Work out the finished part from the listing and answer in its coordinate system (mm). Face numbers are marked on the shaded views. A direction names the side the tool comes from. Coordinates: 2 decimals unless noted, no trailing zeros. Order: outer loops, then holes, each group sorted by start corner. A loop starts at its lowest first (then second) coordinate and runs counter-clockwise, first axis right, second up. Notation, with made-up numbers: (1.5, 54.5) - (20.5, 54.5) arc R13 cw to (20.5, 64.5) - close; hole circle Ø10 at (-20, 62.25). An arc over 180 degrees is marked (long way). Answer as a JSON object with one key per item and string values. Group by question number.
1) Section B-B (x = 2) is taken. Give the vertices of the cut face in (y, z).
2) Each of these flat-tipped pins is pushed along its axis until it touches: P1, Ø0.9, axis at x = -8.5, y = 1, coming from the -Z side; P2, Ø1, axis at x = 4, z = 2, coming from the -Y side; P3, Ø0.9, axis at x = -8.5, y = 0.5, coming from the +Z side. Where does it stop, or does it pass through?
3) Section C-C (y = 1) is taken. Give the vertices of the cut face in (x, z), plus the area to 3 significant figures.
4) A tool of negligible diameter and unlimited length cuts with its end or side. For the marked faces 1 and 2, from which of +Z, -Z, +X, -X, +Y, -Y can it reach the whole face along a straight path? Write none if from no direction.
5) Section A-A (y = 4.25) is taken. Give the vertices of the cut face in (x, z), plus the area to 3 significant figures.
6) Find the intervals of material crossed by line 1 along Z through (x, y) = (1.25, 1.25); line 2 along Z through (x, y) = (6.75, 2); line 3 along Y through (x, z) = (-5.25, 6.25), in increasing order.
7) Section D-D (z = 0.5) is taken. Give the vertices of the cut face in (x, y), plus the area to 3 significant figures.
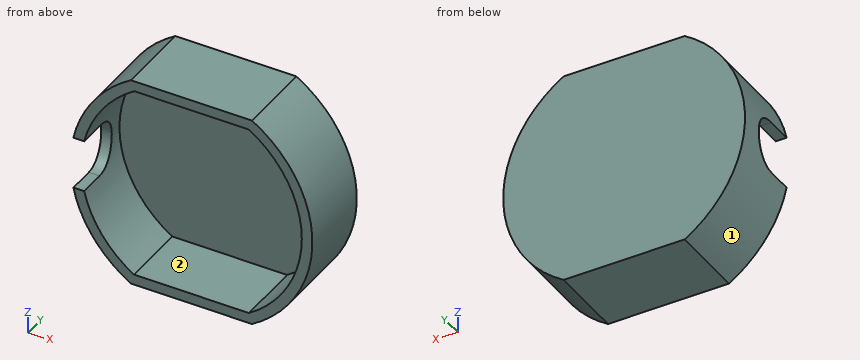
from build123d import *

# Parameters (mm, degrees)
BOSS_EXTRUDE1_DEPTH = 5
BOSS_EXTRUDE2_DEPTH = 0.8
CUT_EXTRUDE1_DEPTH  = 14.556732645


with BuildPart() as part:
    # Sketch1 → Boss-Extrude1 (new body)
    with BuildSketch(Plane(origin=(0, 0, 0), x_dir=(1, 0, 0), z_dir=(0, 1, 0))):
        with BuildLine():
            ThreePointArc((4.577951386, 8.15), (9.15, 0), (4.577951386, -8.15))
            Line((4.577951386, -8.15), (-4.577951386, -8.15))
            ThreePointArc((-4.577951386, -8.15), (-9.15, 0), (-4.577951386, 8.15))
            Line((-4.577951386, 8.15), (4.577951386, 8.15))
        make_face()
        with BuildLine():
            Line((4.347630988, 7.35), (-4.347630988, 7.35))
            ThreePointArc((-4.347630988, 7.35), (-8.35, 0), (-4.347630988, -7.35))
            Line((-4.347630988, -7.35), (4.347630988, -7.35))
            ThreePointArc((4.347630988, -7.35), (8.35, 0), (4.347630988, 7.35))
        make_face(mode=Mode.SUBTRACT)
    extrude(amount=BOSS_EXTRUDE1_DEPTH)

    # Sketch2 → Boss-Extrude2 (add)
    with BuildSketch(Plane(origin=(0, 5, 0), x_dir=(1, 0, 0), z_dir=(0, 1, 0))):
        with BuildLine():
            Line((4.577951386, -8.15), (-4.577951386, -8.15))
            ThreePointArc((-4.577951386, -8.15), (-9.15, 0), (-4.577951386, 8.15))
            Line((-4.577951386, 8.15), (4.577951386, 8.15))
            ThreePointArc((4.577951386, 8.15), (9.15, 0), (4.577951386, -8.15))
        make_face()
    extrude(amount=BOSS_EXTRUDE2_DEPTH)

    # Sketch3 → Cut-Extrude1 (cut, through all)
    with BuildSketch(Plane(origin=(0, 0, 0), x_dir=(0, 0, -1), z_dir=(1, 0, 0))):
        with BuildLine():
            Line((-2, 2), (-2, 0))
            Line((-2, 0), (2, 0))
            Line((2, 0), (2, 2))
            ThreePointArc((2, 2), (0, 4), (-2, 2))
        make_face()
    extrude(amount=-CUT_EXTRUDE1_DEPTH, mode=Mode.SUBTRACT)


solid = part.part
Report:
{
 "1": {"outline": "(0, -8.15) - (5.8, -8.15) - (5.8, 8.15) - (0, 8.15) - (0, 7.35) - (5, 7.35) - (5, -7.35) - (0, -7.35) - close"},
 "2": {"P1": "stops at z = -4.45", "P2": "stops at y = 5", "P3": "stops at z = 4.45"},
 "3": {"outline": "(-8.94, -2) arc R9.55 ccw to (-4.58, -8.15) - (4.58, -8.15) arc R9.55 ccw to (4.58, 8.15) - (-4.58, 8.15) arc R9.55 ccw to (-8.94, 2) - (-8.12, 2) arc R8.75 cw to (-4.35, 7.35) - (4.35, 7.35) arc R8.75 cw to (4.35, -7.35) - (-4.35, -7.35) arc R8.75 cw to (-8.12, -2) - close", "area": "40.6 mm²"},
 "4": {"face 1": "-X, +Y, -Y", "face 2": "-Y"},
 "5": {"outline": "(-4.58, -8.15) - (4.58, -8.15) arc R9.55 ccw to (4.58, 8.15) - (-4.58, 8.15) arc R9.55 ccw to start; hole (-4.35, -7.35) - (4.35, -7.35) arc R8.75 ccw to (4.35, 7.35) - (-4.35, 7.35) arc R8.75 ccw to start", "area": "43.9 mm²"},
 "6": {"line 1": "z = -8.15 to -7.35, 7.35 to 8.15", "line 2": "z = -6.33 to -5.04, 5.04 to 6.33", "line 3": "y = 5 to 5.8"},
 "7": {"outline": "(-9.14, 3.94) - (-8.34, 3.94) - (-8.34, 5) - (8.34, 5) - (8.34, 0) - (9.14, 0) - (9.14, 5.8) - (-9.14, 5.8) - close", "area": "19.5 mm²"}
}
